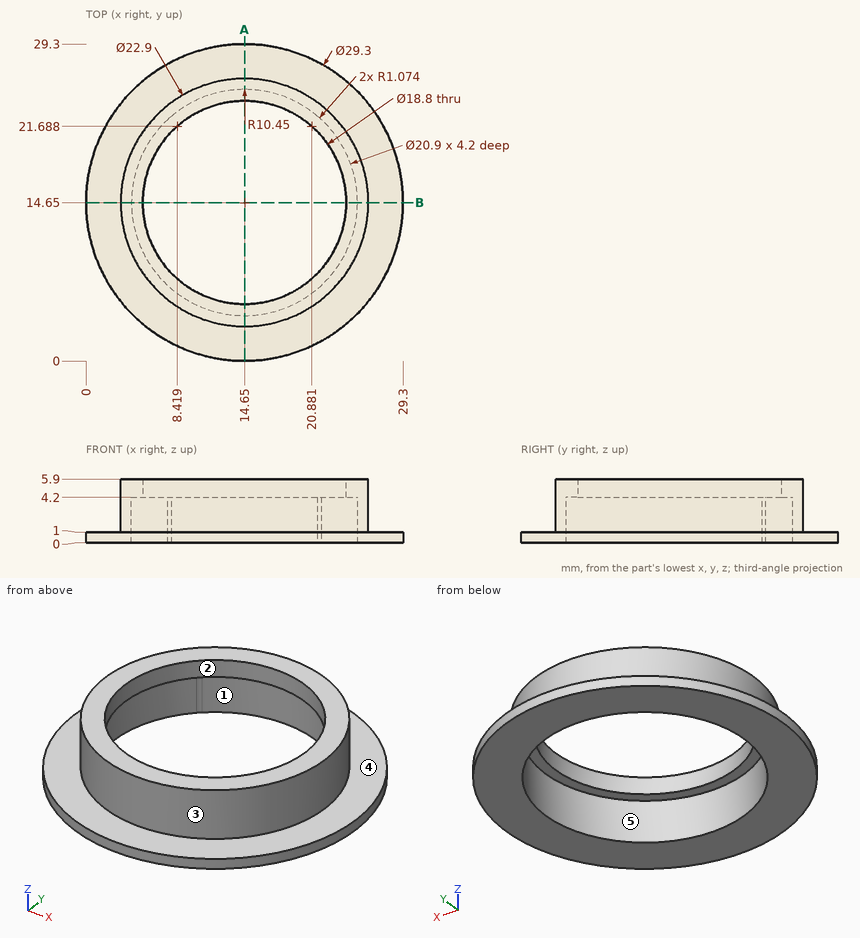
Study the drawing (mm; zero at the part's minimum x, y, z) and answer. A direction names the side the tool comes from. Coordinates: 2 decimals unless noted, no trailing zeros. Write each loop counter-clockwise with the first axis right and the second up, starting at its lowest first coordinate (ties: lowest second). Pieces come first, ordered by that corner, then holes. Notation, with made-up numbers: (29, 89) - (88, 89) arc R36 cw to (88, 128) - close; hole circle Ø9 at (-31, 27). An arc over 180 degrees is marked (long way). Answer as a JSON object with one key per item and string values. Group by question number.
1. Each of these flat-tipped pins is pushed along its axis until it touches: P1, Ø16.5, axis at x = 15, y = 16, coming from the -Z side; P2, Ø2, axis at y = 22, z = 3, coming from the -X side; P3, Ø1.5, axis at y = 5, z = 4.5, coming from the +X side (1 decimal). Where does it stop, or does it pass through?
2. A cutting plane is placed at A-A (x = 14.65). Determine the outline of the cut face in (y, z).
3. Which of the six approach directions +Z, -Z, +X, -X, +Y, -Y give full straight-line access (tool end or side, diameter ignored) to the marked faces 1 and 2?
4. Consider L1, parallel to Y at x = 14.65, z = 4.75; L2, parallel to Y at x = 15, z = 3.45 (1 decimal); L3, parallel to X at y = 10.5, z = 3.95. Determine where each line is inside the solid, lowest interval first. Write a range as [from, to].
5. The mould has two halves that part along X. Classify the marked faces 3, 4 and 5: +X half, -X half, draft (parallel to the pull), parting line (faces both ways), or undercut.
Worked out:
{
 "1": {"P1": "stops at z = 4.2", "P2": "stops at x = 5.12", "P3": "stops at x = 21.9"},
 "2": {"outline": "(0, 0) - (4.2, 0) - (4.2, 4.2) - (5.25, 4.2) - (5.25, 5.9) - (3.2, 5.9) - (3.2, 1) - (0, 1) - close; (24.05, 4.2) - (25.1, 4.2) - (25.1, 0) - (29.3, 0) - (29.3, 1) - (26.1, 1) - (26.1, 5.9) - (24.05, 5.9) - close"},
 "3": {"face 1": "-Z", "face 2": "+Z, -Z"},
 "4": {"L1": "y = [3.2, 5.25], [24.05, 26.1]", "L2": "y = [3.2, 4.2], [25.1, 26.1]", "L3": "x = [3.98, 5.06], [24.24, 25.32]"},
 "5": {"face 3": "parting line", "face 4": "draft", "face 5": "undercut"}
}
